from build123d import *

# Parameters (mm, degrees)
SKETCH_1_W          = 67.3
SKETCH_1_H          = 34
EXTRUDE_1_DEPTH     = 4
SKETCH_2_W          = 21.15
SKETCH_2_H          = 4
EXTRUDE_2_DEPTH     = 42.3
SKETCH_3_W          = 42.3
SKETCH_3_H          = 4
EXTRUDE_3_DEPTH     = 4
FILLET_1_R          = 2
FILLET_2_R          = 2
SKETCH_4_R          = 1.3
SKETCH_4_R_2        = 11.5
CUT_EXTRUDE_1_DEPTH = 4
SKETCH_5_R          = 2.5
CUT_EXTRUDE_2_DEPTH = 4


with BuildPart() as part:
    # Sketch 1 → Extrude 1 (new body)
    with BuildSketch(Plane.XY):
        Rectangle(SKETCH_1_W, SKETCH_1_H)
    extrude(amount=EXTRUDE_1_DEPTH)



with BuildPart() as body_2:
    # Sketch 2 → Extrude 2 (new body)
    with BuildSketch(Plane.XY.offset(4)):
        with Locations((-10.575, 19)):
            Rectangle(SKETCH_2_W, SKETCH_2_H)
        with Locations((10.575, 19)):
            Rectangle(SKETCH_2_W, SKETCH_2_H)
    extrude(amount=EXTRUDE_2_DEPTH)


with BuildPart() as part_1:
    add(part.part)

    add(body_2.part)  # Extrude 3 merges body 2
    # Sketch 3 → Extrude 3 (add)
    with BuildSketch(Plane(origin=(0, 0, 4), x_dir=(-1, 0, 0), z_dir=(0, 0, -1))):
        with Locations((0, 19)):
            Rectangle(SKETCH_3_W, SKETCH_3_H)
    extrude(amount=EXTRUDE_3_DEPTH)

    # Fillet 1
    fillet_1_edges = [part_1.edges().sort_by_distance(p)[0] for p in [
        (0, 17, 4),
    ]]
    fillet(fillet_1_edges, radius=FILLET_1_R)

    # Fillet 2
    fillet_2_edges = [part_1.edges().sort_by_distance(p)[0] for p in [
        (-21.15, 17, 2),
        (21.15, 17, 2),
    ]]
    fillet(fillet_2_edges, radius=FILLET_2_R)

    # Sketch 4 → Cut-Extrude 1 (cut)
    with BuildSketch(Plane.XZ.offset(-17)):
        with Locations((-15.5, 40.65)):
            Circle(SKETCH_4_R)
        with Locations((15.5, 40.65)):
            Circle(SKETCH_4_R)
        with Locations((-15.5, 9.65)):
            Circle(SKETCH_4_R)
        with Locations((15.5, 9.65)):
            Circle(SKETCH_4_R)
        with Locations((0, 25.15)):
            Circle(SKETCH_4_R_2)
    extrude(amount=-CUT_EXTRUDE_1_DEPTH, mode=Mode.SUBTRACT)

    # Sketch 5 → Cut-Extrude 2 (cut)
    with BuildSketch(Plane.XY.offset(4)):
        with Locations((-25.65, 8)):
            Circle(SKETCH_5_R)
        with Locations(Location((-25.65, -8, 0), (0, 0, 180))):
            Circle(SKETCH_5_R)
        with Locations(Location((25.65, 8, 0), (0, 0, 180))):
            Circle(SKETCH_5_R)
        with Locations((25.65, -8)):
            Circle(SKETCH_5_R)
    extrude(amount=-CUT_EXTRUDE_2_DEPTH, mode=Mode.SUBTRACT)


solid = part_1.part
Geometry: final body of the model. Coordinates: model frame, mm. A direction names the side the tool comes from. Round coordinates to 2 decimals unless told otherwise and drop trailing zeros. Order: outer loops, then holes, each group sorted by start corner. A loop starts at its lowest first (then second) coordinate and runs counter-clockwise, first axis right, second up.
Q1. Section A-A, the plane x = -15.5. Output: boundary loops of the cut face in (y, z).
Result sheet:
outline: (-17, 0) - (21, 0) - (21, 8.35) - (17, 8.35) - (17, 6) arc R2 cw to (15, 4) - (-17, 4) - close; (17, 10.95) - (21, 10.95) - (21, 39.35) - (17, 39.35) - close; (17, 41.95) - (21, 41.95) - (21, 46.3) - (17, 46.3) - close
Q2. Section B-B, the plane y = -8. Output: boundary loops of the cut face in (x, z).
Result sheet:
outline: (-33.65, 0) - (-28.15, 0) - (-28.15, 4) - (-33.65, 4) - close; (-23.15, 0) - (23.15, 0) - (23.15, 4) - (-23.15, 4) - close; (28.15, 0) - (33.65, 0) - (33.65, 4) - (28.15, 4) - close
Q3. Material intervals for probe 1 along Z at (x, y) = (15.5, 19.15); probe 2 along Z at (x, y) = (15, 18); probe 3 along Z at (x, y) = (31.5, -6.5), sorted ascending.
Result sheet:
probe 1: z = 0 to 8.35, 10.95 to 39.35, 41.95 to 46.3
probe 2: z = 0 to 8.45, 10.85 to 39.45, 41.85 to 46.3
probe 3: z = 0 to 4
Q4. Pin query (flat end, axial travel): pin 1 (6.5 mm diameter, centred on y = 18, z = 25, fed in from +X); pin 2 (2 mm diameter, centred on x = 29.5, z = 3, fed in from +Y); pin 3 (4 mm diameter, centred on x = -13, z = 29, fed in from -Y). Return the tip coordinate at first contact, or that it passes through.
Result sheet:
pin 1: stops at x = 21.15
pin 2: stops at y = 17
pin 3: stops at y = 17
Q5. Mould query, pull axis X, two halves, no side actions, for faces 6 (the face through (21.72, 17.6, 1.97)), 7 (the face through (0.3, 16.43, 4.6)), 8 (the face through (24.5, 10.22, 2.03)), 9 (the face through (-33.65, 0, 2)). Classes: released by +X, released by -X, zero draft, split by the parting line, or undercut.
Result sheet:
face 6: released by +X
face 7: zero draft
face 8: undercut
face 9: released by -X
Q6. Section C-C, the plane z = 25.15. Output: boundary loops of the cut face in (x, y).
Result sheet:
outline: (-21.15, 17) - (-11.5, 17) - (-11.5, 21) - (-21.15, 21) - close; (11.5, 17) - (21.15, 17) - (21.15, 21) - (11.5, 21) - close
Q7. Section D-D, the plane x = 0. Output: boundary loops of the cut face in (y, z), and give its area (3 significant figures).
Result sheet:
outline: (-17, 0) - (21, 0) - (21, 13.65) - (17, 13.65) - (17, 6) arc R2 cw to (15, 4) - (-17, 4) - close; (17, 36.65) - (21, 36.65) - (21, 46.3) - (17, 46.3) - close
area: 230 mm2
Q8. Access query for faces 1 (the face through (0, -17, 2)), 2 (the face through (-10, 17, 35)), 3 (the face through (-28, 17, 2)), 4 (the face through (-26.8, -5.78, 2.03)), 5 (the face through (28, 17, 2)). Directions: +Z, -Z, +X, -X, +Y, -Y. A direction counts if a zero-diameter tool reaches every point of the face in a straight line with its end or side. Return the directions, or none.
Result sheet:
face 1: +Z, -Z, +X, -X, -Y
face 2: +Z, +X, -X, -Y
face 3: +Z, -Z, -X, +Y
face 4: +Z, -Z
face 5: +Z, -Z, +X, +Y
